Source: CAD feature listing. Evaluate the final solid. Frame: model axes, mm. Coordinates: 2 decimals unless noted, no trailing zeros. Order: outer loops, then holes, each group sorted by start corner. A loop starts at its lowest first (then second) coordinate and runs counter-clockwise, first axis right, second up.
Item 1: Contact query for a flat-ended pin moving along its axis: P1, Ø1.8, axis at x = -45.95, z = -9, coming from the +Y side. Output: stop coordinate, or through.
Item 2: Section A-A on z = 9. Return the cut outline in (x, y).
Item 3: Ray query, line 1 (X direction, y = 1.3, z = 9); line 2 (X direction, y = 1.6, z = 18.5); line 3 (X direction, y = 1.55, z = 29). Return the intervals inside material, ascending.
Item 4: Section B-B on z = -18.5. Return the cut outline in (x, y), then the cut area to 3 significant figures.
from build123d import *

# Parameters (mm, degrees)
ESBO_O1_W                = 100
ESBO_O1_H                = 63
RESSALTO_EXTRUS_O1_DEPTH = 2
ESBO_O5_R                = 2
CORTE_EXTRUS_O3_DEPTH    = 60.129096053
FILETE1_R                = 3
ESBO_O6_R                = 1.15
CORTE_EXTRUS_O4_DEPTH    = 60.129096053


with BuildPart() as part:
    # Esboço1 → Ressalto-extrusão1 (new body)
    with BuildSketch(Plane(origin=(0, 0, 0), x_dir=(1, 0, 0), z_dir=(0, 1, 0))):
        Rectangle(ESBO_O1_W, ESBO_O1_H)
    extrude(amount=RESSALTO_EXTRUS_O1_DEPTH)

    # Esboço5 → Corte-extrusão3 (cut, through all)
    with BuildSketch(Plane(origin=(0, 2, 0), x_dir=(1, 0, 0), z_dir=(0, 1, 0))):
        with Locations(Location((46, 18.5, 0), (0, 0, 270))):
            Circle(ESBO_O5_R)
        with Locations(Location((46, -18.5, 0), (0, 0, 90))):
            Circle(ESBO_O5_R)
        with Locations(Location((-46, -18.5, 0), (0, 0, 270))):
            Circle(ESBO_O5_R)
        with Locations(Location((-46, 18.5, 0), (0, 0, 90))):
            Circle(ESBO_O5_R)
    extrude(amount=-CORTE_EXTRUS_O3_DEPTH, mode=Mode.SUBTRACT)

    # Filete1
    filete1_edges = [part.edges().sort_by_distance(p)[0] for p in [
        (-50, 1, -31.5),
        (50, 1, -31.5),
        (50, 1, 31.5),
        (-50, 1, 31.5),
    ]]
    fillet(filete1_edges, radius=FILETE1_R)

    # Esboço6 → Corte-extrusão4 (cut, through all)
    with BuildSketch(Plane.XZ):
        with Locations(Location((45.95, 9, 0), (0, 0, 270))):
            Circle(ESBO_O6_R)
        with Locations(Location((45.95, -9, 0), (0, 0, 90))):
            Circle(ESBO_O6_R)
        with Locations(Location((-45.95, -9, 0), (0, 0, 270))):
            Circle(ESBO_O6_R)
        with Locations(Location((-45.95, 9, 0), (0, 0, 90))):
            Circle(ESBO_O6_R)
    extrude(amount=-CORTE_EXTRUS_O4_DEPTH, mode=Mode.SUBTRACT)


solid = part.part
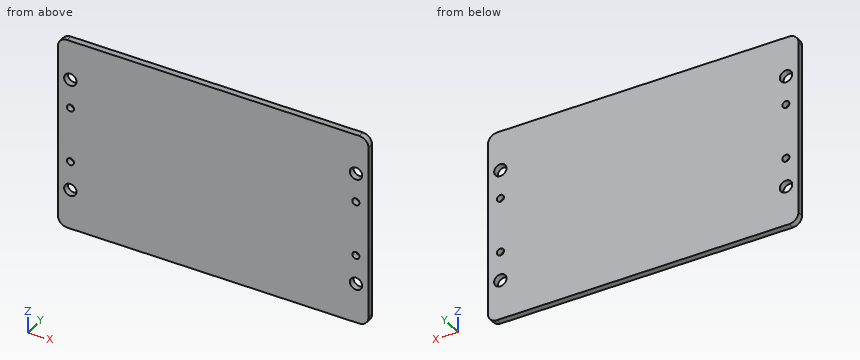
Answer list:
1. P1: passes through
2. outline: (-50, 0) - (-47.1, 0) - (-47.1, 2) - (-50, 2) - close; (-44.8, 0) - (44.8, 0) - (44.8, 2) - (-44.8, 2) - close; (47.1, 0) - (50, 0) - (50, 2) - (47.1, 2) - close
3. line 1: x = -50 to -47.1, -44.8 to 44.8, 47.1 to 50
3. line 2: x = -50 to -48, -44 to 44, 48 to 50
3. line 3: x = -49.96 to 49.96
4. outline: (-50, 0) - (-48, 0) - (-48, 2) - (-50, 2) - close; (-44, 0) - (44, 0) - (44, 2) - (-44, 2) - close; (48, 0) - (50, 0) - (50, 2) - (48, 2) - close
4. area: 184 mm2
